Could you check a few things on this drawing? It's one solid part, dimensions in mm from its lowest x, y, z. Give positions to 0.01 mm unless a question says otherwise; leave off trailing zeros. Loops run counter-clockwise (first coordinate to the right, second up) from the corner with the lowest first, then second, coordinate; pieces in that order, holes last. Notation, with made-up numbers: M -10,-9 L 41,-9 A17 cw 41,15 Z; hole C 27,-6.75 d4. An arc over 180 degrees is marked long. Return JSON: item names as keys, results as strings. Group by question number.
1. For pin 1 (12 mm diameter, centred on x = 38.5, y = 9.5, fed in from -Z); pin 2 (2.5 mm diameter, centred on x = 362, z = 21.5, fed in from +Y); pin 3 (2.5 mm diameter, centred on x = 359.5, z = 21, fed in from -Y), each with a flat end and sliding along its axis, tell me the tip position at first contact or that it passes through.
2. If we section it at B-B (z = 22.5): Write out the boundary of the cut face in (x, y), plus the area to 3 significant figures.
3. Please list where these lines run through material, in increasing order: line 1 (Y direction, x = 26, z = 23); line 2 (X direction, y = 22.75, z = 16.25); line 3 (X direction, y = 18.75, z = 3.75).
4. If we section it at C-C (y = 21.75): Write out the boundary of the cut face in (x, z).
5. If we section it at D-D (x = 136): Write out the boundary of the cut face in (y, z), plus the area to 3 significant figures.
6. If we section it at A-A (y = 3): Write out the boundary of the cut face in (x, z), plus the area to 3 significant figures.
7. If we mould it in two halves opening along X, with no side actions, what happens to the marked faces 1 and 2? For each: +X half, -X half, draft (parallel to the pull), parting line (faces both ways), or undercut.
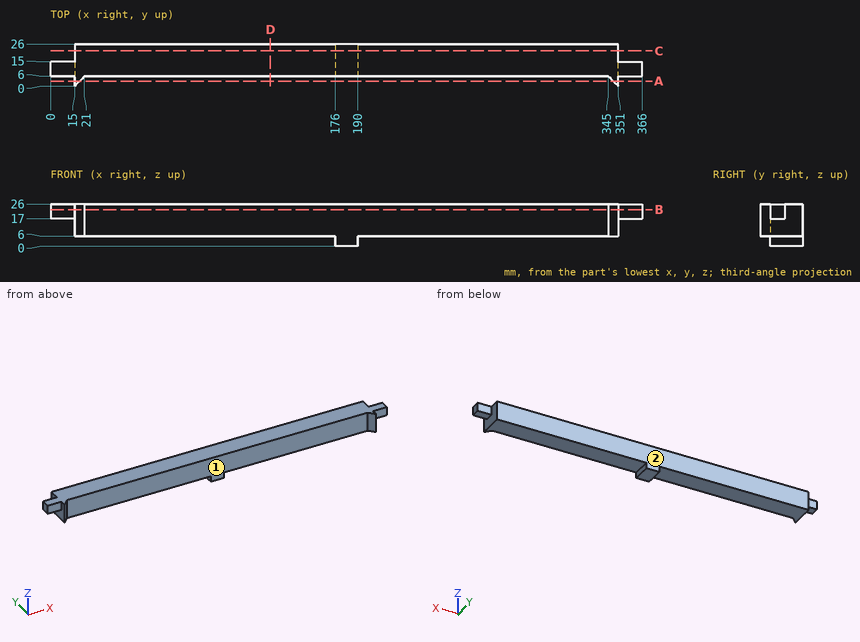
Answer:
{
 "1": {"pin 1": "stops at z = 6", "pin 2": "stops at y = 15", "pin 3": "stops at y = 6"},
 "2": {"outline": "M 0,6 L 15,6 L 15,0 L 21,6 L 345,6 L 351,0 L 351,6 L 366,6 L 366,15 L 351,15 L 351,26 L 15,26 L 15,15 L 0,15 Z", "area": "7,030 mm²"},
 "3": {"line 1": "y = 6 to 26", "line 2": "x = 15 to 351", "line 3": "x = 176 to 190"},
 "4": {"outline": "M 15,6 L 176,6 L 176,0 L 190,0 L 190,6 L 351,6 L 351,26 L 15,26 Z"},
 "5": {"outline": "M 6,6 L 26,6 L 26,26 L 6,26 Z", "area": "400 mm²"},
 "6": {"outline": "M 15,6 L 18,6 L 18,26 L 15,26 Z; M 348,6 L 351,6 L 351,26 L 348,26 Z", "area": "120 mm²"},
 "7": {"face 1": "undercut", "face 2": "draft"}
}
